Part model, mm, in its own coordinate system. A direction names the side the tool comes from. Coordinates: 2 decimals unless noted, no trailing zeros. Loops run counter-clockwise (first coordinate to the right, second up) from the corner with the lowest first, then second, coordinate; pieces in that order, holes last. Notation, with made-up numbers: (27.5, 33) -> (61.5, 33) arc R23 cw to (61.5, 52) -> close; hole circle Ø11 at (-25.75, 20). An arc over 180 degrees is marked (long way). One line per question, with ' | ' between items. Start each with the question number.
1) Drop flat-ended pins along their axis: pin 1 (2 mm diameter, centred on x = -7, y = 10, fed in from +Z); pin 2 (12 mm diameter, centred on x = -10.5, y = 22, fed in from +Z); pin 3 (12 mm diameter, centred on x = 13, z = 42, fed in from -Y); pin 4 (1.5 mm diameter, centred on x = -22.5, z = 7, fed in from +Y). Give the stop position or say it passes through.
2) Cut at A-A (z = 39.5). List the corners of the cut face in (x, y), plus the area to 3 significant figures.
3) Two-plate mould, pull along X, no slides. Class faces 3 (the face through (0, -2, 25.4)), 4 (the face through (-9.153, -12.871, 37.421)), 5 (the face through (15, 23.53, 12.52)), 6 (the face through (21, 13, 25.4)): released by +X, released by -X, zero draft, split by the parting line, or undercut.
4) Cut at D-D (z = 17). List the corners of the cut face in (x, y).
5) Probe L1, parallel to Z at x = 2, y = 4.5; L2, parallel to X at y = 5.5, z = 46.5; L3, parallel to Y at x = -3, z = 35.5. List the from-to ranges inside material, lowest first. Write a range as from..to.
6) 3-axis set-ups, long thin cutter, end or side, ignore diameter. For faces 1 (the face through (0, 0, 0)), 2 (the face through (-3.106, 23.658, 37.421)): which of +Z, -Z, +X, -X, +Y, -Y reach the whole face in a straight line?
7) Cut at C-C (x = 12.5). List the corners of the cut face in (y, z).
8) Cut at B-B (y = 0). List the corners of the cut face in (x, z) (3 decimals), plus the area to 3 significant figures.
from build123d import *

# Parameters (mm, degrees)
F0_R     = 27.903603
F1_DEPTH = 25.4
F2_R     = 23.860723
F3_DEPTH = 24.384


with BuildPart() as f1:
    # F0 (on Top) → F1 (new body)
    with BuildSketch(Plane.XY):
        Circle(F0_R)
    extrude(amount=F1_DEPTH)

    # F2 (on face) → F3 (join)
    with BuildSketch(Plane.XY.offset(25.4)):
        Circle(F2_R)
        Polygon((-18.564959, -6.032121), (-11.473776, 15.792297), (11.473776, 15.792297), (18.564959, -6.032121), (0, -19.520353), align=None, mode=Mode.SUBTRACT)
    extrude(amount=F3_DEPTH)


solid = f1.part
Reported:
1) pin 1: stops at z = 25.4 | pin 2: stops at z = 49.78 | pin 3: stops at y = -22.81 | pin 4: stops at y = 17.48
2) outline: circle Ø47.72 at (0, 0); hole (-18.56, -6.03) -> (0, -19.52) -> (18.56, -6.03) -> (11.47, 15.79) -> (-11.47, 15.79) -> close | area: 883 mm²
3) face 3: undercut | face 4: undercut | face 5: split by the parting line | face 6: zero draft
4) outline: circle Ø55.81 at (0, 0)
5) L1: z = 0..25.4 | L2: x = -23.22..-14.82, 14.82..23.22 | L3: y = -23.67..-17.34, 15.79..23.67
6) face 1: -Z, +X, -X, +Y, -Y | face 2: +Z
7) outline: (-24.95, 0) -> (24.95, 0) -> (24.95, 25.4) -> (20.32, 25.4) -> (20.32, 49.78) -> (12.63, 49.78) -> (12.63, 25.4) -> (-10.44, 25.4) -> (-10.44, 49.78) -> (-20.32, 49.78) -> (-20.32, 25.4) -> (-24.95, 25.4) -> close
8) outline: (-27.904, 0) -> (27.904, 0) -> (27.904, 25.4) -> (23.861, 25.4) -> (23.861, 49.784) -> (16.605, 49.784) -> (16.605, 25.4) -> (-16.605, 25.4) -> (-16.605, 49.784) -> (-23.861, 49.784) -> (-23.861, 25.4) -> (-27.904, 25.4) -> close | area: 1,770 mm²
